Design review of the part built by this model. Coordinates are the model's own, in mm. Face numbers are marked on the shaded views. A direction names the side the tool comes from. Give positions to 0.01 mm unless a question says otherwise; leave off trailing zeros. Order: outer loops, then holes, each group sorted by start corner. A loop starts at its lowest first (then second) coordinate and runs counter-clockwise, first axis right, second up.
```python
from build123d import *

# Parameters (mm, degrees)
F1_DEPTH = 5
F3_DEPTH = 15
F5_DEPTH = 25


with BuildPart() as f1:
    # F0 (on Top) → F1 (new body)
    with BuildSketch(Plane.XY):
        with BuildLine():
            Line((-13.163356, 15.594428), (-16.72976, 6.733515))
            ThreePointArc((-16.72976, 6.733515), (0, -18.033999), (16.72976, 6.733515))
            Line((16.72976, 6.733515), (13.173763, 15.568571))
            Line((13.173763, 15.568571), (9.308094, 6.733515))
            Line((9.308094, 6.733515), (-7.921782, 6.733515))
            Line((-7.921782, 6.733515), (-13.163356, 15.594428))
        make_face()
    extrude(amount=F1_DEPTH)

    # F2 (on face) → F3 (cut)
    with BuildSketch(Plane.XY.offset(5)):
        Polygon((-13.163356, 11.163971), (-14.946558, 6.822401), (-10.915843, 6.733515), align=None)
    extrude(amount=-F3_DEPTH, mode=Mode.SUBTRACT)

    # F4 (on face) → F5 (cut)
    with BuildSketch(Plane.XY.offset(5)):
        Polygon((13.173763, 11.151043), (11.305694, 6.733515), (15.009284, 6.733515), align=None)
    extrude(amount=-F5_DEPTH, mode=Mode.SUBTRACT)


solid = f1.part
```
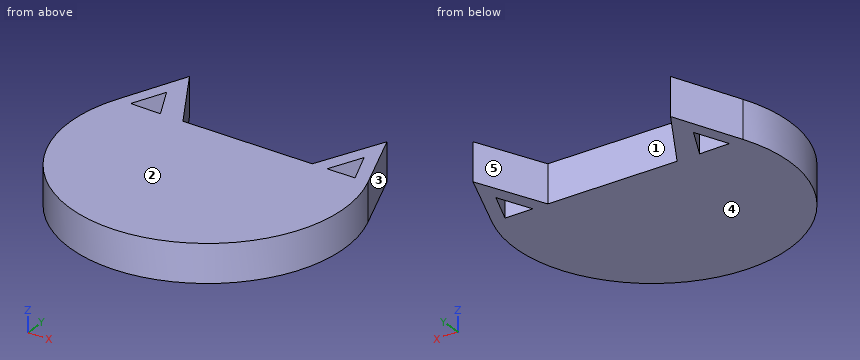
1. Take a section at B-B (x = 14). State the section outline as (y, z) points.
Recorded:
outline: (-11.37, 0) - (6.73, 0) - (6.73, 5) - (-11.37, 5) - close; (9.16, 0) - (13.52, 0) - (13.52, 5) - (9.16, 5) - close
2. Machinability: for the marked faces 1 and 2, which of the approach directions +Z, -Z, +X, -X, +Y, -Y give a long, thin tool a straight path to every point of the face, cutting with its end or side? Answer none if there is none.
Recorded:
face 1: +Z, -Z, +Y
face 2: +Z, +X, -X, +Y, -Y
3. Draft analysis for pull direction X (two halves, no side actions). For the marked faces 3, 4 and 5, state which applies: pulls with the +X half, pulls with the -X half, needs draft (parallel to the pull), parting line crosses it, or undercut.
Recorded:
face 3: pulls with the +X half
face 4: needs draft
face 5: undercut
4. Take a section at C-C (y = 13). State the section outline as (x, z) points, then the cut area to 3 significant figures.
Recorded:
outline: (-14.21, 0) - (-11.63, 0) - (-11.63, 5) - (-14.21, 5) - close; (12.05, 0) - (14.21, 0) - (14.21, 5) - (12.05, 5) - close
area: 23.7 mm2
5. Take a section at A-A (z = 2.05). State the section outline as (x, y) points, then the cut area to 3 significant figures.
Recorded:
outline: (-16.73, 6.73) arc R18.03 ccw (long way) to (16.73, 6.73) - (13.17, 15.57) - (9.31, 6.73) - (-7.92, 6.73) - (-13.16, 15.59) - close; hole (-14.95, 6.82) - (-10.92, 6.73) - (-13.16, 11.16) - close; hole (11.31, 6.73) - (15.01, 6.73) - (13.17, 11.15) - close
area: 803 mm2
6. For pin 1 (1 mm diameter, centred on x = 6, z = 3.5, fed in from +Y); pin 2 (1.5 mm diameter, centred on y = 10, z = 3, fed in from +X); pin 3 (3 mm diameter, centred on x = 13.5, z = 1.5, fed in from +Y), all flat-tipped, find the tip position at first contact; note any pin that passes through.
Recorded:
pin 1: stops at y = 6.73
pin 2: stops at x = 15.72
pin 3: stops at y = 15.57
7. For line 1 along X through (y, z) = (9.5, 3.6); line 2 along X through (y, z) = (0, 1); line 3 along Y through (x, z) = (-11, 2.3), list the stretches that pass through material, from the lowest coordinate up.
Recorded:
line 1: x = -15.62 to -13.85, -12.32 to -9.56, 10.52 to 12.48, 13.86 to 15.62
line 2: x = -18.03 to 18.03
line 3: y = -14.29 to 6.74, 6.9 to 11.94
8. Take a section at D-D (x = 0). State the section outline as (y, z) points.
Recorded:
outline: (-18.03, 0) - (6.73, 0) - (6.73, 5) - (-18.03, 5) - close
